from build123d import *

# Parameters (mm, degrees)
SKETCH_1_W                       = 44
SKETCH_1_H                       = 50
SKETCH_1_R                       = 2
SM_BASE_FLANGE_1_DEPTH           = 3
SM_EDGE_FLANGE_1_STRIP_W         = 13.4732
SM_EDGE_FLANGE_1_STRIP_H         = 3
SM_EDGE_FLANGE_1_STRIP_CUT_DEPTH = 50
SM_EDGE_FLANGE_1_DEPTH           = 50
SM_EDGE_FLANGE_2_STRIP_W         = 13.4732
SM_EDGE_FLANGE_2_STRIP_H         = 3
SM_EDGE_FLANGE_2_STRIP_CUT_DEPTH = 50
SM_EDGE_FLANGE_2_DEPTH           = 50
SKETCH_15_R                      = 15
SKETCH_15_R_2                    = 1.5
CUT_EXTRUDE_1_DEPTH              = 3
SKETCH_16_R                      = 1.6
SKETCH_16_R_2                    = 17
CUT_EXTRUDE_2_DEPTH              = 3
CUT_EXTRUDE_5_DEPTH              = 3
SKETCH_18_R                      = 1.6
CUT_EXTRUDE_6_DEPTH              = 3
FILLET_2_R                       = 3
CUT_EXTRUDE_7_DEPTH              = 10


# Sheet-metal steps are written as plain solids
with BuildPart() as part:
    # Sketch 1 → 基体-法兰1 (new body)
    with BuildSketch(Plane(origin=(0, 0, 0), x_dir=(1, 0, 0), z_dir=(0, 1, 0))):
        with Locations((-2, 0)):
            Rectangle(SKETCH_1_W, SKETCH_1_H)
        with Locations(Location((0, 12, 0), (0, 0, 270))):
            Circle(SKETCH_1_R, mode=Mode.SUBTRACT)
        with Locations(Location((10.392304845, 6, 0), (0, 0, 270))):
            Circle(SKETCH_1_R, mode=Mode.SUBTRACT)
        with Locations(Location((10.392304845, -6, 0), (0, 0, 270))):
            Circle(SKETCH_1_R, mode=Mode.SUBTRACT)
        with Locations(Location((0, -12, 0), (0, 0, 270))):
            Circle(SKETCH_1_R, mode=Mode.SUBTRACT)
        with Locations(Location((-10.392304845, -6, 0), (0, 0, 270))):
            Circle(SKETCH_1_R, mode=Mode.SUBTRACT)
        with Locations(Location((-10.392304845, 6, 0), (0, 0, 270))):
            Circle(SKETCH_1_R, mode=Mode.SUBTRACT)
    extrude(amount=-SM_BASE_FLANGE_1_DEPTH)

    # 边线-法兰1 strip (across the edge) → 边线-法兰1 strip cut (cut)
    with BuildSketch(Plane(origin=(20, -3, -25), x_dir=(-1, 0, 0), z_dir=(0, 0, 1))):
        with Locations((-6, -1.5)):
            Rectangle(SM_EDGE_FLANGE_1_STRIP_W, SM_EDGE_FLANGE_1_STRIP_H)
    extrude(amount=SM_EDGE_FLANGE_1_STRIP_CUT_DEPTH, mode=Mode.SUBTRACT)

    # 边线-法兰1 section (across the edge) → 边线-法兰1 (add)
    with BuildSketch(Plane(origin=(20, -3, -25), x_dir=(-1, 0, 0), z_dir=(0, 0, 1))):
        with BuildLine():
            Line((-3, 0.7366), (-3, 57))
            Line((-3, 57), (0, 57))
            Line((0, 57), (0, 0.7366))
            ThreePointArc((0, 0.7366), (0.215745145, 0.215745145), (0.7366, 0))
            Line((0.7366, 0), (0.7366, -3))
            ThreePointArc((0.7366, -3), (-1.905575199, -1.905575199), (-3, 0.7366))
        make_face()
    extrude(amount=SM_EDGE_FLANGE_1_DEPTH)

    # 边线-法兰2 strip (across the edge) → 边线-法兰2 strip cut (cut)
    with BuildSketch(Plane(origin=(-24, -3, 25), x_dir=(1, 0, 0), z_dir=(0, 0, -1))):
        with Locations((-6, -1.5)):
            Rectangle(SM_EDGE_FLANGE_2_STRIP_W, SM_EDGE_FLANGE_2_STRIP_H)
    extrude(amount=SM_EDGE_FLANGE_2_STRIP_CUT_DEPTH, mode=Mode.SUBTRACT)

    # 边线-法兰2 section (across the edge) → 边线-法兰2 (add)
    with BuildSketch(Plane(origin=(-24, -3, 25), x_dir=(1, 0, 0), z_dir=(0, 0, -1))):
        with BuildLine():
            Line((-3, 0.7366), (-3, 57))
            Line((-3, 57), (0, 57))
            Line((0, 57), (0, 0.7366))
            ThreePointArc((0, 0.7366), (0.215745145, 0.215745145), (0.7366, 0))
            Line((0.7366, 0), (0.7366, -3))
            ThreePointArc((0.7366, -3), (-1.905575199, -1.905575199), (-3, 0.7366))
        make_face()
    extrude(amount=SM_EDGE_FLANGE_2_DEPTH)

    # 草图15 → 切除-拉伸1 (cut)
    with BuildSketch(Plane.ZY.offset(27)):
        with Locations(Location((0, -35, 0), (0, 0, 270))):
            Circle(SKETCH_15_R)
        with Locations(Location((0, -15.75, 0), (0, 0, 270))):
            Circle(SKETCH_15_R_2)
        with Locations(Location((19.25, -35, 0), (0, 0, 270))):
            Circle(SKETCH_15_R_2)
        with Locations(Location((0, -54.25, 0), (0, 0, 270))):
            Circle(SKETCH_15_R_2)
        with Locations(Location((-19.25, -35, 0), (0, 0, 270))):
            Circle(SKETCH_15_R_2)
    extrude(amount=-CUT_EXTRUDE_1_DEPTH, mode=Mode.SUBTRACT)

    # 草图16 → 切除-拉伸2 (cut)
    with BuildSketch(Plane(origin=(23, 0, 0), x_dir=(0, 0, -1), z_dir=(1, 0, 0))):
        with Locations(Location((17.878805079, -24.468578969, 0), (0, 0, 90))):
            Circle(SKETCH_16_R)
        with Locations(Location((20.089063538, -40.195385084, 0), (0, 0, 90))):
            Circle(SKETCH_16_R)
        with Locations(Location((10.531421031, -52.878805079, 0), (0, 0, 90))):
            Circle(SKETCH_16_R)
        with BuildLine():
            ThreePointArc((-3.595385084, -55.089063538), (-4.993466734, -53.501855618), (-6.744421309, -54.688455531))
            ThreePointArc((-6.744421309, -54.688455531), (-5.595993091, -56.638099762), (-3.64634886, -55.489671544))
            ThreePointArc((-3.64634886, -55.489671544), (-3.608177165, -55.290981888), (-3.595385084, -55.089063538))
        make_face()
        with Locations(Location((-17.878805079, -45.531421031, 0), (0, 0, 90))):
            Circle(SKETCH_16_R)
        with Locations(Location((-20.089063538, -29.804614916, 0), (0, 0, 90))):
            Circle(SKETCH_16_R)
        with Locations(Location((-10.531421031, -17.121194921, 0), (0, 0, 90))):
            Circle(SKETCH_16_R)
        with Locations(Location((5.195385084, -14.910936462, 0), (0, 0, 90))):
            Circle(SKETCH_16_R)
        with Locations(Location((0, -35, 0), (0, 0, 90))):
            Circle(SKETCH_16_R_2)
    extrude(amount=-CUT_EXTRUDE_2_DEPTH, mode=Mode.SUBTRACT)

    # 草图17 → 切除-拉伸5 (cut)
    with BuildSketch(Plane.ZY.offset(27)):
        with BuildLine():
            ThreePointArc((0, -50), (-6.123724357, -48.693063938), (-11.180339887, -45))
            ThreePointArc((-11.180339887, -45), (-18.623701364, -43.974644577), (-25, -40))
            Line((-25, -40), (-25, -60))
            Line((-25, -60), (0, -60))
            Line((0, -60), (0, -55.75))
            ThreePointArc((0, -55.75), (-1.5, -54.25), (0, -52.75))
            Line((0, -52.75), (0, -50))
        make_face()
        with BuildLine():
            Line((25, -60), (25, -40))
            ThreePointArc((25, -40), (18.623701364, -43.974644577), (11.180339887, -45))
            ThreePointArc((11.180339887, -45), (6.123724357, -48.693063938), (0, -50))
            Line((0, -50), (0, -52.75))
            ThreePointArc((0, -52.75), (1.060660172, -53.189339828), (1.5, -54.25))
            ThreePointArc((1.5, -54.25), (1.060660172, -55.310660172), (0, -55.75))
            Line((0, -55.75), (0, -60))
            Line((0, -60), (25, -60))
        make_face()
        with BuildLine():
            ThreePointArc((15, -35), (10.606601718, -24.393398282), (0, -20))
            Line((0, -20), (0, -45))
            Line((0, -45), (11.180339887, -45))
            ThreePointArc((11.180339887, -45), (14.012585384, -40.352331347), (15, -35))
        make_face()
        with BuildLine():
            Line((0, -45), (0, -20))
            ThreePointArc((0, -20), (-13.693063938, -28.876275643), (-11.180339887, -45))
            Line((-11.180339887, -45), (0, -45))
        make_face()
        with BuildLine():
            Line((11.180339887, -45), (0, -45))
            Line((0, -45), (0, -50))
            ThreePointArc((0, -50), (6.123724357, -48.693063938), (11.180339887, -45))
        make_face()
        with BuildLine():
            Line((0, -50), (0, -45))
            Line((0, -45), (-11.180339887, -45))
            ThreePointArc((-11.180339887, -45), (-6.123724357, -48.693063938), (0, -50))
        make_face()
    extrude(amount=-CUT_EXTRUDE_5_DEPTH, mode=Mode.SUBTRACT)

    # 草图18 → 切除-拉伸6 (cut)
    # profile 1 of 5: a face of its own
    with BuildSketch(Plane(origin=(23, 0, 0), x_dir=(0, 0, -1), z_dir=(1, 0, 0))):
        with BuildLine():
            ThreePointArc((13.743814378, -45.005376871), (0, -52), (-13.743814378, -45.005376871))
            ThreePointArc((-13.743814378, -45.005376871), (-15.17808001, -44.848040907), (-16.595135856, -44.576332908))
            ThreePointArc((-16.595135856, -44.576332908), (-16.359945185, -45.028365745), (-16.278805079, -45.531421031))
            ThreePointArc((-16.278805079, -45.531421031), (-18.786243203, -46.849205555), (-18.449500144, -44.036661137))
            ThreePointArc((-18.449500144, -44.036661137), (-21.942963359, -42.372436612), (-25, -40))
            Line((-25, -40), (-25, -60))
            Line((-25, -60), (25, -60))
            Line((25, -60), (25, -40))
            ThreePointArc((25, -40), (19.81343454, -43.495603445), (13.743814378, -45.005376871))
        make_face()
        with Locations((-5.195385084, -55.089063538)):
            Circle(SKETCH_18_R, mode=Mode.SUBTRACT)
        with Locations((10.531421031, -52.878805079)):
            Circle(SKETCH_18_R, mode=Mode.SUBTRACT)
    # profile 2 of 5: a face of its own
    with BuildSketch(Plane(origin=(23, 0, 0), x_dir=(0, 0, -1), z_dir=(1, 0, 0))):
        with BuildLine():
            Line((11.180339887, -45), (-11.180339887, -45))
            ThreePointArc((-11.180339887, -45), (-12.461981292, -45.048381264), (-13.743814378, -45.005376871))
            ThreePointArc((-13.743814378, -45.005376871), (0, -52), (13.743814378, -45.005376871))
            ThreePointArc((13.743814378, -45.005376871), (12.461981292, -45.048381264), (11.180339887, -45))
        make_face()
    # profile 3 of 5: a face of its own
    with BuildSketch(Plane(origin=(23, 0, 0), x_dir=(0, 0, -1), z_dir=(1, 0, 0))):
        with BuildLine():
            ThreePointArc((-16.595135856, -44.576332908), (-15.17808001, -44.848040907), (-13.743814378, -45.005376871))
            ThreePointArc((-13.743814378, -45.005376871), (-15.519532338, -41.938596112), (-16.620858499, -38.570302896))
            ThreePointArc((-16.620858499, -38.570302896), (-21.118873978, -36.850650515), (-25, -34))
            Line((-25, -34), (-25, -40))
            ThreePointArc((-25, -40), (-21.942963359, -42.372436612), (-18.449500144, -44.036661137))
            ThreePointArc((-18.449500144, -44.036661137), (-17.431709516, -43.995157526), (-16.595135856, -44.576332908))
        make_face()
    # profile 4 of 5: a face of its own
    with BuildSketch(Plane(origin=(23, 0, 0), x_dir=(0, 0, -1), z_dir=(1, 0, 0))):
        with BuildLine():
            ThreePointArc((-13.743814378, -45.005376871), (-12.461981292, -45.048381264), (-11.180339887, -45))
            Line((-11.180339887, -45), (11.180339887, -45))
            ThreePointArc((11.180339887, -45), (12.461981292, -45.048381264), (13.743814378, -45.005376871))
            ThreePointArc((13.743814378, -45.005376871), (15.519532338, -41.938596112), (16.620858499, -38.570302896))
            ThreePointArc((16.620858499, -38.570302896), (13.916978953, -38.992540305), (11.180339887, -39))
            Line((11.180339887, -39), (-11.180339887, -39))
            ThreePointArc((-11.180339887, -39), (-13.916978953, -38.992540305), (-16.620858499, -38.570302896))
            ThreePointArc((-16.620858499, -38.570302896), (-15.519532338, -41.938596112), (-13.743814378, -45.005376871))
        make_face()
    # profile 5 of 5: a face of its own
    with BuildSketch(Plane(origin=(23, 0, 0), x_dir=(0, 0, -1), z_dir=(1, 0, 0))):
        with BuildLine():
            ThreePointArc((16.620858499, -38.570302896), (15.519532338, -41.938596112), (13.743814378, -45.005376871))
            ThreePointArc((13.743814378, -45.005376871), (19.81343454, -43.495603445), (25, -40))
            Line((25, -40), (25, -34))
            ThreePointArc((25, -34), (21.118873978, -36.850650515), (16.620858499, -38.570302896))
        make_face()
        with Locations((20.089063538, -40.195385084)):
            Circle(SKETCH_18_R, mode=Mode.SUBTRACT)
    extrude(amount=-CUT_EXTRUDE_6_DEPTH, mode=Mode.SUBTRACT)

    # 圆角2
    fillet_2_edges = [part.edges().sort_by_distance(p)[0] for p in [
        (-25.5, -45, 11.180339887),
        (-25.5, -45, -11.180339887),
        (21.5, -38.570302896, -16.620858499),
        (21.5, -38.570302896, 16.620858499),
    ]]
    fillet(fillet_2_edges, radius=FILLET_2_R)

    # 草图19 → 切除-拉伸7 (cut)
    with BuildSketch(Plane.ZY.offset(27)):
        with BuildLine():
            Line((-7.5, -5.5), (7.5, -5.5))
            ThreePointArc((7.5, -5.5), (10.5, -8.5), (7.5, -11.5))
            Line((7.5, -11.5), (-7.5, -11.5))
            ThreePointArc((-7.5, -11.5), (-10.5, -8.5), (-7.5, -5.5))
        make_face()
    extrude(amount=-CUT_EXTRUDE_7_DEPTH, mode=Mode.SUBTRACT)


solid = part.part
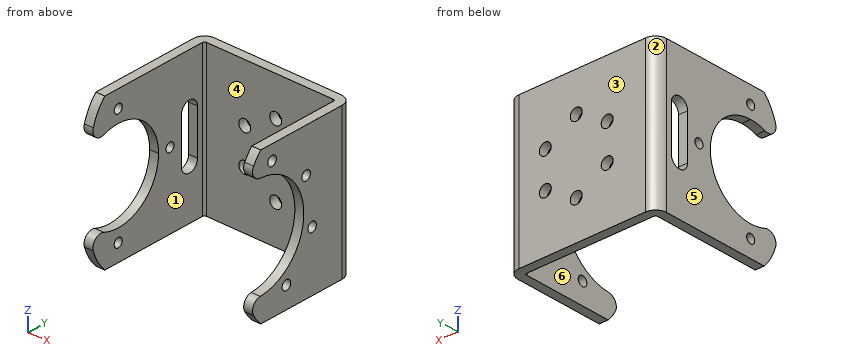
Here's how the part is built. I have some questions about the finished solid (model axes, mm). Face numbers are marked on the shaded views. A direction names the side the tool comes from. Coordinates: 2 decimals unless noted, no trailing zeros. Loops run counter-clockwise (first coordinate to the right, second up) from the corner with the lowest first, then second, coordinate; pieces in that order, holes last.
1. I need wall thicknesses on L1, parallel to X at y = -12.5, z = 21; L2, parallel to X at y = -1, z = -12; L3, parallel to Y at x = -19, z = -2.5. Which ranges of each line are inside material? Lowest first, please.
2. If we mould it in two halves opening along X, with no side actions, what happens to the marked faces 1, 2, 3 and 4? For each: pulls with the +X half, pulls with the -X half, needs draft (parallel to the pull), parting line crosses it, or undercut.
3. Imagine slicing it at C-C, the plane z = -12. Please give me the cut outline in (x, y), and give its area (3 significant figures).
4. Imagine slicing it at A-A, the plane x = 0. Please give me the cut outline in (y, z), and give its area (3 significant figures).
5. For the marked faces 5 and 6, which set-ups out of +Z, -Z, +X, -X, +Y, -Y let a thin tool reach every point of the face, with its end or its side?
6. For P1, Ø3.5, axis at x = -26, z = -1.5, coming from the +Y side; P2, Ø13, axis at x = 6.5, z = -8, coming from the -Y side; P3, Ø16.5, axis at y = -24.5, z = 9, coming from the -X side; P4, Ø2.5, axis at x = -25, z = -1, coming from the -Y side, each with a flat end and sliding along its axis, tell me the tip position at first contact or that it passes through.
7. Imagine slicing it at D-D, the plane y = -22. Please give me the cut outline in (x, z).
8. Imagine slicing it at B-B, the plane y = -8.5. Please give me the cut outline in (x, z), and give its area (3 significant figures).
Taken from the geometry:
1. L1: x = -27 to -24, 20 to 23
1. L2: x = -25.81 to -2, 2 to 21.81
1. L3: y = -3 to 0
2. face 1: undercut
2. face 2: pulls with the -X half
2. face 3: needs draft
2. face 4: undercut
3. outline: (-27, -26) - (-24, -26) - (-24, -3.74) arc R0.74 cw to (-23.26, -3) - (-2, -3) - (-2, 0) - (-23.26, 0) arc R3.74 ccw to (-27, -3.74) - close; (2, -3) - (19.26, -3) arc R0.74 cw to (20, -3.74) - (20, -22.96) - (23, -22.96) - (23, -3.74) arc R3.74 ccw to (19.26, 0) - (2, 0) - close
3. area: 261 mm2
4. outline: (-3, -25) - (0, -25) - (0, -14) - (-3, -14) - close; (-3, -10) - (0, -10) - (0, 10) - (-3, 10) - close; (-3, 14) - (0, 14) - (0, 25) - (-3, 25) - close
4. area: 126 mm2
5. face 5: +Z, -Z, -X, +Y, -Y
5. face 6: +Z, -Z, -Y
6. P1: stops at y = -0.13
6. P2: stops at y = -3
6. P3: stops at x = -27
6. P4: stops at y = -20.17
7. outline: (-27, -25) - (-24, -25) - (-24, -7.48) - (-27, -7.48) - close; (-27, 7.48) - (-24, 7.48) - (-24, 25) - (-27, 25) - close; (20, -25) - (23, -25) - (23, -10.95) - (20, -10.95) - close; (20, 10.95) - (23, 10.95) - (23, 25) - (20, 25) - close
8. outline: (-27, -25) - (-24, -25) - (-24, -10.5) - (-27, -10.5) - close; (-27, 10.5) - (-24, 10.5) - (-24, 25) - (-27, 25) - close; (20, -25) - (23, -25) - (23, 25) - (20, 25) - close
8. area: 237 mm2
